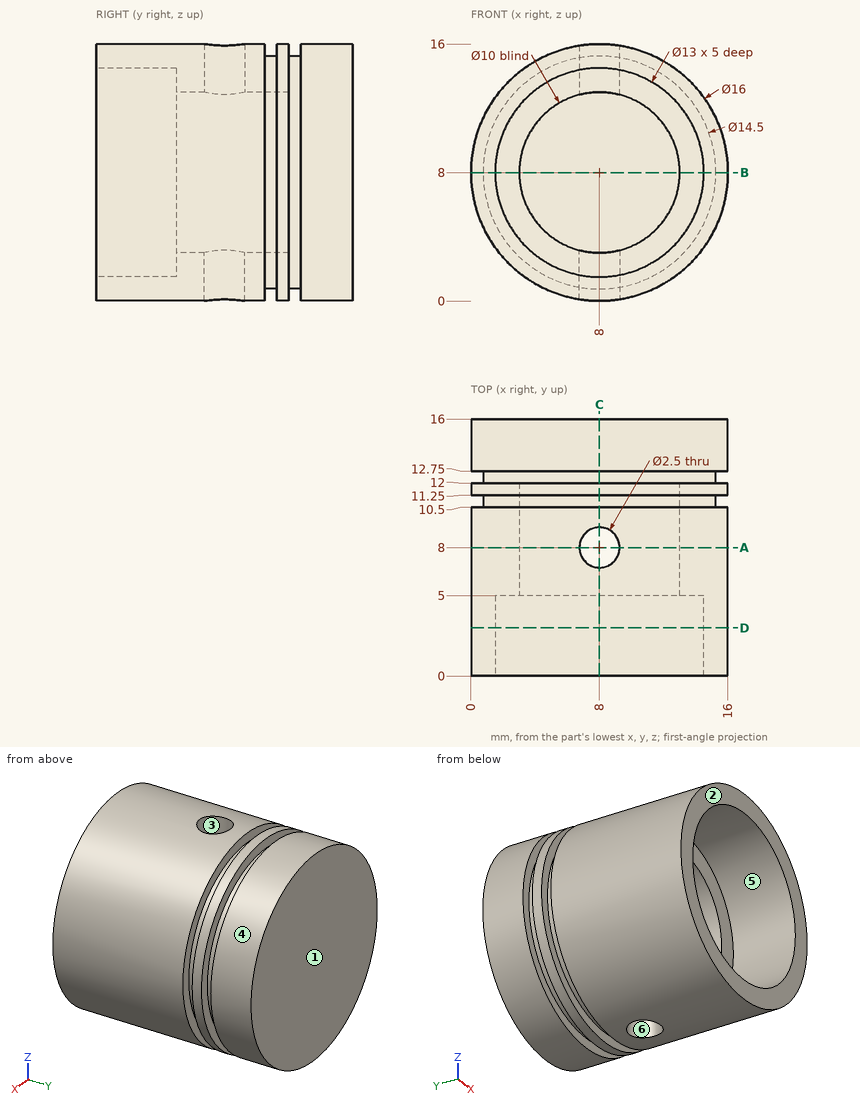
Geometry check sheet. Reference: drawing and pictorial views, mm from the part's lowest x, y, z. A direction names the side the tool comes from. Give positions to 0.01 mm unless a question says otherwise; leave off trailing zeros. Write each loop counter-clockwise with the first axis right and the second up, starting at its lowest first coordinate (ties: lowest second). Pieces come first, ordered by that corner, then holes.
Item 1: Cross-section at C-C (x = 8). Count the separate pieces of the cut face and the enclosed holes in it, and give its area (3 significant figures).
Item 2: Scan lines: L1, parallel to Y at x = 8, z = 1.55; L2, parallel to Y at x = 2.25, z = 2.5; L3, parallel to Z at x = 8, y = 1. Record each from-to range of solid material in increasing order.
Item 3: Draft check along Y on the marked faces 1, 2, 3 and 4. Enter one of: released by +Y, released by -Y, zero draft, split by the parting line, or undercut.
Item 4: Cross-section at A-A (y = 8). Enter the section's corners in (x, z).
Item 5: Access from +Z, -Z, +X, -X, +Y, -Y to the whole of each face (thin tool, end or side, straight path). Record for the marked faces 5 and 6.
Item 6: Cross-section at D-D (y = 3). Enter the section's corners in (x, z), and give its area (3 significant figures).
Item 7: Gauge pin test, flat ends, axial feed: pin 1 (1 mm diameter, centred on y = 4, z = 13.5, fed in from -X) (3 decimals); pin 2 (3 mm diameter, centred on x = 8, y = 8, fed in from +Z); pin 3 (4 mm diameter, centred on x = 7, z = 10.5, fed in from -Y); pin 4 (4 mm diameter, centred on x = 10.5, z = 10, fed in from -Y). Record the tip position at first contact, or that the pin passes through.
Item 8: Cross-section at B-B (z = 8). Enter the section's corners in (x, y).
Report:
1. separate pieces: 3
1. enclosed holes: 0
1. area: 104 mm2
2. L1: y = 5 to 6.75, 9.25 to 16
2. L2: y = 0 to 10.5, 11.25 to 12, 12.75 to 16
2. L3: z = 0 to 1.5, 14.5 to 16
3. face 1: released by +Y
3. face 2: released by -Y
3. face 3: undercut
3. face 4: zero draft
4. outline: (6.75, 0.1) - (6.75, 3.16) arc R5 cw to (6.75, 12.84) - (6.75, 15.9) arc R8 ccw to start; (9.25, 0.1) arc R8 ccw to (9.25, 15.9) - (9.25, 12.84) arc R5 cw to (9.25, 3.16) - close
5. face 5: -Y
5. face 6: +Z, -Z
6. outline: circle Ø16 at (8, 8); hole circle Ø13 at (8, 8)
6. area: 68.3 mm2
7. pin 1: stops at x = 1.755
7. pin 2: stops at z = 16
7. pin 3: stops at y = 12
7. pin 4: stops at y = 5
8. outline: (0, 0) - (1.5, 0) - (1.5, 5) - (3, 5) - (3, 12) - (13, 12) - (13, 5) - (14.5, 5) - (14.5, 0) - (16, 0) - (16, 10.5) - (15.25, 10.5) - (15.25, 11.25) - (16, 11.25) - (16, 12) - (15.25, 12) - (15.25, 12.75) - (16, 12.75) - (16, 16) - (0, 16) - (0, 12.75) - (0.75, 12.75) - (0.75, 12) - (0, 12) - (0, 11.25) - (0.75, 11.25) - (0.75, 10.5) - (0, 10.5) - close
